from build123d import *

# Parameters (mm, degrees)
SKETCH1_R           = 3.4925
BOSS_EXTRUDE1_DEPTH = 3.8227


with BuildPart() as part:
    # Sketch1 → Boss-Extrude1 (new body, symmetric)
    with BuildSketch(Plane(origin=(0, 0, 0), x_dir=(1, 0, 0), z_dir=(0, 1, 0))):
        Circle(SKETCH1_R)
        Polygon((1.374815329, -2.38125), (2.749630657, 0), (1.374815329, 2.38125), (-1.374815329, 2.38125), (-2.749630657, 0), (-1.374815329, -2.38125), align=None, mode=Mode.SUBTRACT)
    extrude(amount=BOSS_EXTRUDE1_DEPTH, both=True)


solid = part.part
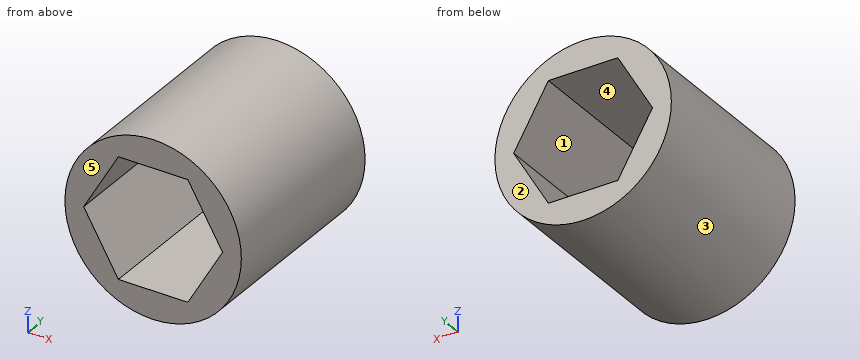
Read the model definition and answer for the solid it produces. Units are mm, in the model's axes. Face numbers are marked on the shaded views. A direction names the side the tool comes from. Give positions to 0.01 mm unless a question says otherwise; leave off trailing zeros. Write each loop counter-clockwise with the first axis right and the second up, starting at its lowest first coordinate (ties: lowest second). Pieces come first, ordered by that corner, then holes. Notation, with made-up numbers: (22, 49.5) - (71, 49.5) arc R10 cw to (71, 57.5) - close; hole circle Ø6 at (-26, 20). An arc over 180 degrees is marked (long way). Answer in a Markdown table with one row per item. Add a question column.
Item 1: Section B-B, the plane x = 0 is taken. Write down the section's boundary in (y, z), and give its area (3 significant figures).
Item 2: Determine the mould class of the marked faces 3, 4 and 5 for opening direction X: pulls with the +X half, pulls with the -X half, needs draft (parallel to the pull), parting line crosses it, or undercut.
Item 3: Section C-C, the plane z = -1.75 is taken. Write down the section's boundary in (x, y), and give its area (3 significant figures).
Item 4: Find the intervals of material crossed by L1, parallel to Z at x = 0.5, y = 0.75; L2, parallel to Z at x = -2.25, y = 3.25; L3, parallel to X at y = 3.5, z = 1.75, in increasing order.
Item 5: Section D-D, the plane z = 3 is taken. Write down the section's boundary in (x, y).
Item 6: Section A-A, the plane y = 2 is taken. Write down the section's boundary in (x, z) (1 decimal).
Item 7: A tool of negligible diameter and unlimited length cuts with its end or side. For the marked faces 1 and 2, from which of +Z, -Z, +X, -X, +Y, -Y can it reach the whole face along a straight path? Write none if from no direction.
Item 8: Flat-ended cylindrical pins translate along their axes: P1, Ø3, axis at y = 1.5, z = 3, coming from the -X side; P2, Ø2, axis at x = -1.5, y = 1, coming from the -Z side; P3, Ø1, axis at x = -2, y = -1, coming from the -Z side. Find the tip coordinate at first contact, or state that the pin passes through.
Recorded:
| question | item | result |
|---|---|---|
| 1 | outline | (-3.82, -3.49) - (3.82, -3.49) - (3.82, -2.38) - (-3.82, -2.38) - close; (-3.82, 2.38) - (3.82, 2.38) - (3.82, 3.49) - (-3.82, 3.49) - close |
| 1 | area | 17.0 mm2 |
| 2 | face 3 | parting line crosses it |
| 2 | face 4 | undercut |
| 2 | face 5 | needs draft |
| 3 | outline | (-3.02, -3.82) - (-1.74, -3.82) - (-1.74, 3.82) - (-3.02, 3.82) - close; (1.74, -3.82) - (3.02, -3.82) - (3.02, 3.82) - (1.74, 3.82) - close |
| 3 | area | 19.6 mm2 |
| 4 | L1 | z = -3.46 to -2.38, 2.38 to 3.46 |
| 4 | L2 | z = -2.67 to -0.87, 0.87 to 2.67 |
| 4 | L3 | x = -3.02 to -1.74, 1.74 to 3.02 |
| 5 | outline | (-1.79, -3.82) - (1.79, -3.82) - (1.79, 3.82) - (-1.79, 3.82) - close |
| 6 | outline | circle Ø7 at (0, 0); hole (-2.7, 0) - (-1.4, -2.4) - (1.4, -2.4) - (2.7, 0) - (1.4, 2.4) - (-1.4, 2.4) - close |
| 7 | face 1 | +Y, -Y |
| 7 | face 2 | +Z, -Z, +X, -X, +Y |
| 8 | P1 | stops at x = -3.15 |
| 8 | P2 | stops at z = -3.46 |
| 8 | P3 | stops at z = -3.15 |
